Could you check a few things on this drawing? It's one solid part, dimensions in mm from its lowest x, y, z. Round coordinates to 2 decimals unless told otherwise and drop trailing zeros. Order: outer loops, then holes, each group sorted by start corner. A loop starts at its lowest first (then second) coordinate and runs counter-clockwise, first axis right, second up. Notation, with made-up numbers: (-26, -3.5) - (-21, -3.5) arc R22 ccw to (-21, 15.5) - close; hole circle Ø1 at (-32.5, 19.5). An arc over 180 degrees is marked (long way). Use one line per item in the form item = value.
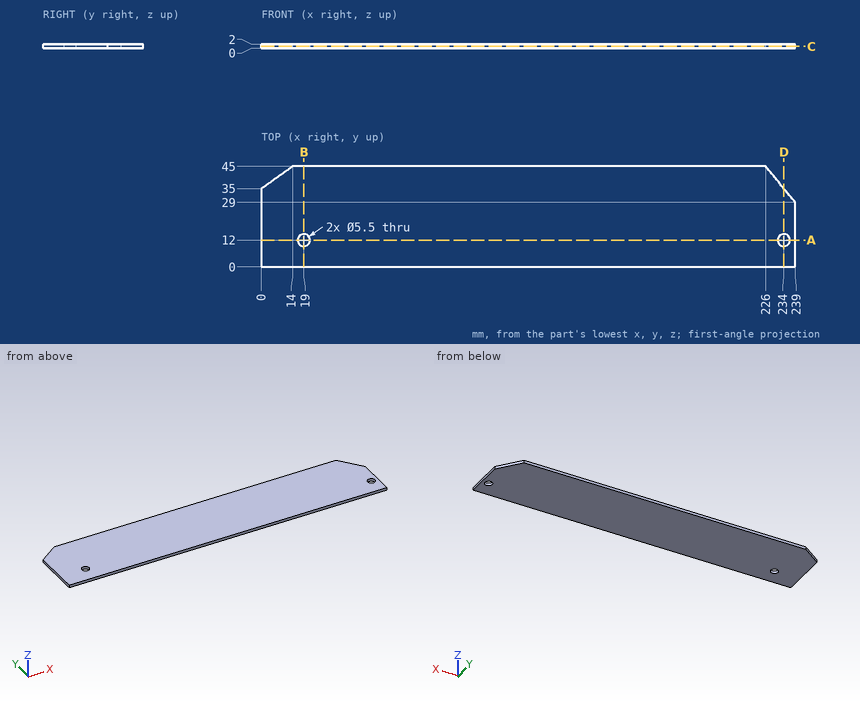
Item 1: Imagine slicing it at C-C on z = 0.9. Please give me the cut outline in (x, y).
Found:
outline = (0, 0) - (239, 0) - (239, 29) - (226, 45) - (14, 45) - (0, 35) - close; hole circle Ø5.5 at (19, 12); hole circle Ø5.5 at (234, 12)
Item 2: Imagine slicing it at B-B on x = 19. Please give me the cut outline in (y, z), plus the area to 3 significant figures.
Found:
outline = (0, 0) - (9.25, 0) - (9.25, 2) - (0, 2) - close; (14.75, 0) - (45, 0) - (45, 2) - (14.75, 2) - close
area = 79.0 mm2
Item 3: Imagine slicing it at D-D on x = 234. Please give me the cut outline in (y, z).
Found:
outline = (0, 0) - (9.25, 0) - (9.25, 2) - (0, 2) - close; (14.75, 0) - (35.15, 0) - (35.15, 2) - (14.75, 2) - close
Item 4: I need wall thicknesses on L1, parallel to Y at x = 19, z = 1.1; L2, parallel to Y at x = 234, z = 1.1; L3, parallel to X at y = 40, z = 1.9. Which ranges of each line are inside material? Lowest first, please.
Found:
L1 = 0 to 9.25, 14.75 to 45
L2 = 0 to 9.25, 14.75 to 35.15
L3 = 7 to 230.06
Item 5: Imagine slicing it at A-A on y = 12. Please give me the cut outline in (x, z).
Found:
outline = (0, 0) - (16.25, 0) - (16.25, 2) - (0, 2) - close; (21.75, 0) - (231.25, 0) - (231.25, 2) - (21.75, 2) - close; (236.75, 0) - (239, 0) - (239, 2) - (236.75, 2) - close
